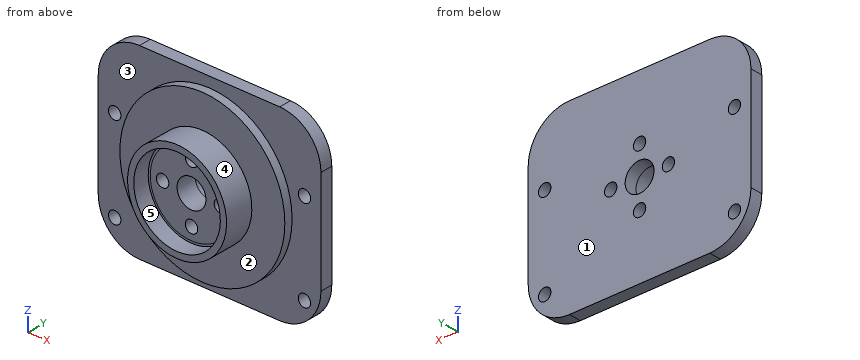
```python
from build123d import *
from build123d.topology import SkipClean

# Parameters (mm, degrees)
SKETCH_1_W      = 54
SKETCH_1_H      = 45
SKETCH_1_R      = 1.5
SKETCH_1_R_2    = 3.5
EXTRUDE_1_DEPTH = 3
EXTRUDE_START   = 5
SKETCH_2_R      = 10
SKETCH_2_R_2    = 1.5
SKETCH_2_R_3    = 3.5
EXTRUDE_2_DEPTH = 5
FILLET_1_R      = 10
SKETCH_6_R      = 12
SKETCH_6_R_2    = 10
EXTRUDE_3_DEPTH = 5
EXTRUDE_START_2 = 4
SKETCH_7_R      = 12
SKETCH_7_R_2    = 10.5
EXTRUDE_4_DEPTH = 4
EXTRUDE_START_3 = 2
SKETCH_8_R      = 20
SKETCH_8_R_2    = 12
EXTRUDE_5_DEPTH = 2


with BuildPart() as part:
    # 草图1 → 凸台-拉伸1 (new body)
    with BuildSketch(Plane(origin=(0, 0, 0), x_dir=(1, 0, 0), z_dir=(0, 1, 0))):
        Rectangle(SKETCH_1_W, SKETCH_1_H)
        with Locations(Location((0, 7, 0), (0, 0, 270))):
            Circle(SKETCH_1_R, mode=Mode.SUBTRACT)
        with Locations(Location((7, 0, 0), (0, 0, 270))):
            Circle(SKETCH_1_R, mode=Mode.SUBTRACT)
        with Locations(Location((0, 0, 0), (0, 0, 270))):
            Circle(SKETCH_1_R_2, mode=Mode.SUBTRACT)
        with Locations(Location((0, -7, 0), (0, 0, 90))):
            Circle(SKETCH_1_R, mode=Mode.SUBTRACT)
        with Locations(Location((-7, 0, 0), (0, 0, 90))):
            Circle(SKETCH_1_R, mode=Mode.SUBTRACT)
        with Locations(Location((23, 16, 0), (0, 0, 270))):
            Circle(SKETCH_1_R, mode=Mode.SUBTRACT)
        with Locations(Location((23, -6, 0), (0, 0, 90))):
            Circle(SKETCH_1_R, mode=Mode.SUBTRACT)
        with Locations(Location((-23, -6, 0), (0, 0, 270))):
            Circle(SKETCH_1_R, mode=Mode.SUBTRACT)
        with Locations(Location((-23, 16, 0), (0, 0, 90))):
            Circle(SKETCH_1_R, mode=Mode.SUBTRACT)
    extrude(amount=EXTRUDE_1_DEPTH)

    # 草图2 → 凸台-拉伸2 (add)
    with SkipClean():  # the faces are left unmerged after this step: merging them gives an invalid solid
        with BuildSketch(Plane.XZ.offset(EXTRUDE_START)):
            with Locations(Location((0, 0, 0), (0, 0, 270))):
                Circle(SKETCH_2_R)
            with Locations(Location((0, 7, 0), (0, 0, 270))):
                Circle(SKETCH_2_R_2, mode=Mode.SUBTRACT)
            with Locations(Location((0, 0, 0), (0, 0, 270))):
                Circle(SKETCH_2_R_3, mode=Mode.SUBTRACT)
            with Locations(Location((-7, 0, 0), (0, 0, 270))):
                Circle(SKETCH_2_R_2, mode=Mode.SUBTRACT)
            with Locations(Location((0, -7, 0), (0, 0, 270))):
                Circle(SKETCH_2_R_2, mode=Mode.SUBTRACT)
            with Locations(Location((7, 0, 0), (0, 0, 270))):
                Circle(SKETCH_2_R_2, mode=Mode.SUBTRACT)
        extrude(amount=-EXTRUDE_2_DEPTH)

    # 圆角1
    fillet_1_edges = [part.edges().sort_by_distance(p)[0] for p in [
        (27, 1.5, 22.5),
        (-27, 1.5, 22.5),
        (-27, 1.5, -22.5),
        (27, 1.5, -22.5),
    ]]
    fillet(fillet_1_edges, radius=FILLET_1_R)

    # 草图6 → 凸台-拉伸3 (add)
    with SkipClean():  # the faces are left unmerged after this step: merging them gives an invalid solid
        with BuildSketch(Plane.XZ.offset(EXTRUDE_START)):
            with Locations(Location((0, 0, 0), (0, 0, 270))):
                Circle(SKETCH_6_R)
            Circle(SKETCH_6_R_2, mode=Mode.SUBTRACT)
        extrude(amount=-EXTRUDE_3_DEPTH)

    # 草图7 → 凸台-拉伸4 (add)
    with SkipClean():  # the faces are left unmerged after this step: merging them gives an invalid solid
        with BuildSketch(Plane.XZ.offset(5).offset(EXTRUDE_START_2)):
            with Locations(Location((0, 0, 0), (0, 0, 270))):
                Circle(SKETCH_7_R)
            with Locations(Location((0, 0, 0), (0, 0, 270))):
                Circle(SKETCH_7_R_2, mode=Mode.SUBTRACT)
        extrude(amount=-EXTRUDE_4_DEPTH)

    # 草图8 → 凸台-拉伸5 (add)
    with SkipClean():  # the faces are left unmerged after this step: merging them gives an invalid solid
        with BuildSketch(Plane.XZ.offset(EXTRUDE_START_3)):
            with Locations(Location((0, 0, 0), (0, 0, 270))):
                Circle(SKETCH_8_R)
            with Locations(Location((0, 0, 0), (0, 0, 270))):
                Circle(SKETCH_8_R_2, mode=Mode.SUBTRACT)
        extrude(amount=-EXTRUDE_5_DEPTH)


solid = part.part
```
For this review, take the finished solid that the model builds, in its own axes (mm). Face numbers are marked on the shaded views. A direction names the side the tool comes from. Round coordinates to 2 decimals unless told otherwise and drop trailing zeros. Loops run counter-clockwise (first coordinate to the right, second up) from the corner with the lowest first, then second, coordinate; pieces in that order, holes last.
Q1. Add section A-A on x = 0. Write out the cut boundary in (y, z), plus the area to 3 significant figures.
Result sheet:
outline: (-9, -12) - (-2, -12) - (-2, -20) - (0, -20) - (0, -22.5) - (3, -22.5) - (3, -8.5) - (-5, -8.5) - (-5, -10.5) - (-9, -10.5) - close; (-9, 10.5) - (-5, 10.5) - (-5, 8.5) - (3, 8.5) - (3, 22.5) - (0, 22.5) - (0, 20) - (-2, 20) - (-2, 12) - (-9, 12) - close; (-5, -5.5) - (3, -5.5) - (3, -3.5) - (-5, -3.5) - close; (-5, 3.5) - (3, 3.5) - (3, 5.5) - (-5, 5.5) - close
area: 195 mm2
Q2. Mouldability with a two-part tool opening along X and no side actions: class the marked faces 3, 4 and 5 as +X half, -X half, draft (parallel to the pull), parting line (faces both ways), or undercut.
Result sheet:
face 3: draft
face 4: parting line
face 5: undercut
Q3. Add section C-C on x = -23. Write out the cut boundary in (y, z), plus the area to 3 significant figures.
Result sheet:
outline: (0, -20.5) - (3, -20.5) - (3, -17.5) - (0, -17.5) - close; (0, -14.5) - (3, -14.5) - (3, 4.5) - (0, 4.5) - close; (0, 7.5) - (3, 7.5) - (3, 20.5) - (0, 20.5) - close
area: 105 mm2
Q4. To check wall thickness, follow line 1 along X through (y, z) = (1.55, 0); line 2 along X through (y, z) = (-1.6, 0); line 3 along Z through (x, y) = (0, 1.15). State the ranges of each line that lie inside material, in increasing order.
Result sheet:
line 1: x = -27 to -8.5, -5.5 to -3.5, 3.5 to 5.5, 8.5 to 27
line 2: x = -20 to -8.5, -5.5 to -3.5, 3.5 to 5.5, 8.5 to 20
line 3: z = -22.5 to -8.5, -5.5 to -3.5, 3.5 to 5.5, 8.5 to 22.5
Q5. Machinability: for the marked faces 1 and 2, which of the approach directions +Z, -Z, +X, -X, +Y, -Y give a long, thin tool a straight path to every point of the face, cutting with its end or side? Answer none if there is none.
Result sheet:
face 1: +Z, -Z, +X, -X, +Y
face 2: -Y
Q6. Add section B-B on z = 0. Write out the cut boundary in (x, y).
Result sheet:
outline: (-27, 0) - (-20, 0) - (-20, -2) - (-12, -2) - (-12, -9) - (-10.5, -9) - (-10.5, -5) - (-8.5, -5) - (-8.5, 3) - (-27, 3) - close; (-5.5, -5) - (-3.5, -5) - (-3.5, 3) - (-5.5, 3) - close; (3.5, -5) - (5.5, -5) - (5.5, 3) - (3.5, 3) - close; (8.5, -5) - (10.5, -5) - (10.5, -9) - (12, -9) - (12, -2) - (20, -2) - (20, 0) - (27, 0) - (27, 3) - (8.5, 3) - close
Q7. Add section D-D on y = -1. Write out the cut boundary in (x, z), plus the area to 3 significant figures.
Result sheet:
outline: circle Ø40 at (0, 0); hole circle Ø3 at (-7, 0); hole circle Ø7 at (0, 0); hole circle Ø3 at (0, -7); hole circle Ø3 at (0, 7); hole circle Ø3 at (7, 0)
area: 1,190 mm2
Q8. Insertion check: pin 1 Ø17 at (x, z) = (-4.5, 1) entering from -Y; pin 2 Ø1 at (x, z) = (13.5, -1.5) entering from -Y; pin 3 Ø16 at (x, z) = (1, 2) entering from -Y; pin 4 Ø3 at (y, z) = (1.5, -14.5) entering from +X. Each pin has a flat end and moves straight along its axis. Give the tip position at first contact, or say it passes through.
Result sheet:
pin 1: stops at y = -9
pin 2: stops at y = -2
pin 3: stops at y = -5
pin 4: stops at x = 26.99
